Geometry: final body of the model. Coordinates: model frame, mm. A direction names the side the tool comes from. Give positions to 0.01 mm unless a question says otherwise; leave off trailing zeros. Write each loop counter-clockwise with the first axis right and the second up, starting at its lowest first coordinate (ties: lowest second). Pieces come first, ordered by that corner, then holes.
from build123d import *

# Parameters (mm, degrees)
SKETCH_2_W       = 5
SKETCH_2_H       = 6
SKETCH_2_W_2     = 6
SKETCH_2_H_2     = 5
F_02_SLOTS_DEPTH = 8


with BuildPart() as part:
    # 草图1 → 01_RING (revolve)
    with BuildSketch(Plane.XY, mode=Mode.PRIVATE) as f_01_ring_sk:
        Polygon((0, 17.5), (0, 23), (1, 24), (6, 24), (7, 23), (7, 17.5), align=None)
    revolve(f_01_ring_sk.sketch.rotate(Axis((-5, 0, 0), (1, 0, 0)), 90), axis=Axis((-5, 0, 0), (1, 0, 0)))

    # 草图2 → 02_SLOTS (cut)
    with BuildSketch(Plane(origin=(-0.5, 0, 0), x_dir=(0, 0, -1), z_dir=(1, 0, 0))):
        with Locations((23.5, 0)):
            Rectangle(SKETCH_2_W, SKETCH_2_H)
        with Locations((-23.5, 0)):
            Rectangle(SKETCH_2_W, SKETCH_2_H)
        with Locations((0, 23.5)):
            Rectangle(SKETCH_2_W_2, SKETCH_2_H_2)
        with Locations((0, -23.5)):
            Rectangle(SKETCH_2_W_2, SKETCH_2_H_2)
    extrude(amount=F_02_SLOTS_DEPTH, mode=Mode.SUBTRACT)


solid = part.part
Q1. Pull-direction query (Z, two-part tool) for faces 5 (the flat face through (3, 22, -3)), 6 (the conical face through (6.84, -16.53, -16.22)), 7 (the cylindrical face through (3.54, 17.13, 16.81)); classes: released by +Z, released by -Z, zero draft, split by the parting line, or undercut.
Filled sheet:
face 5: undercut
face 6: released by -Z
face 7: released by +Z
Q2. Ray query, line 1 along Y through (x, z) = (3, 0); line 2 along Y through (x, z) = (1.75, -12.5); line 3 along Z through (x, y) = (2.25, 6). Return the intervals inside material, ascending.
Filled sheet:
line 1: y = -21 to -17.5, 17.5 to 21
line 2: y = -20.49 to -12.25, 12.25 to 20.49
line 3: z = -23.24 to -16.44, 16.44 to 23.24
Q3. Section C-C on x = 5. Output: boundary loops of the cut face in (y, z).
Filled sheet:
outline: (-23.81, -3) arc R24 ccw to (-3, -23.81) - (-3, -21) - (3, -21) - (3, -23.81) arc R24 ccw to (23.81, -3) - (21, -3) - (21, 3) - (23.81, 3) arc R24 ccw to (3, 23.81) - (3, 21) - (-3, 21) - (-3, 23.81) arc R24 ccw to (-23.81, 3) - (-21, 3) - (-21, -3) - close; hole circle Ø35 at (0, 0)
Q4. Section A-A on y = 0. Output: boundary loops of the cut face in (x, z), plus the area to 3 significant figures.
Filled sheet:
outline: (0, -21) - (7, -21) - (7, -17.5) - (0, -17.5) - close; (0, 17.5) - (7, 17.5) - (7, 21) - (0, 21) - close
area: 49.0 mm2
Q5. Access query for faces 1 (the cylindrical face through (3.451, 17.084, -3.794)), 2 (the flat face through (3, 0, -21)), 3 (the flat face through (3, -21, 0)), 4 (the flat face through (3, 0, 21)). Directions: +Z, -Z, +X, -X, +Y, -Y. A direction counts if a zero-diameter tool reaches every point of the face in a straight line with its end or side. Return the directions, or none.
Filled sheet:
face 1: +X, -X
face 2: -Z, +X, -X
face 3: +X, -X, -Y
face 4: +Z, +X, -X
Q6. Pin query (flat end, axial travel): P1, Ø1.4, axis at x = 2, y = 22, coming from the -Z side; P2, Ø2, axis at x = 4, y = 22, coming from the +Z side; P3, Ø4, axis at x = 2, z = 13, coming from the +Y side; P4, Ø5, axis at y = -3.5, z = 18, coming from the -X side. Return the tip coordinate at first contact, or that it passes through.
Filled sheet:
P1: stops at z = -11.06
P2: stops at z = 11.62
P3: stops at y = 21.33
P4: stops at x = 0
